Autodesk Inventor part; units mm, degrees
ref_plane "YZ Plane" through (0, 0, 0) normal (1, 0, 0) x (0, 1, 0)
ref_plane "XZ Plane" through (0, 0, 0) normal (0, 1, 0) x (-1, 0, 0)
ref_plane "XY Plane" through (0, 0, 0) normal (0, 0, 1) x (1, 0, 0)
sketch "Boceto1" plane through (0, 0, 0) normal (0, 0, 1) x (1, 0, 0)
  line L0 (-49.9, -20) -> (-45, -20)
  line L1 (-47.8393, -13.9) -> (-45, -13.9)
  line L2 (-50.5, -16.5607) -> (-47.8393, -13.9)
  line L3 (-50.5, -18.2) -> (-50.5, -16.5607)
  line L4 (-48.1, -18.2) -> (-50.5, -18.2)
  line L5 (-49.9, -20) -> (-48.1, -18.2)
  line L6 (-55, -20) -> (-45, -20)
  line L7 (-55, -5.1) -> (-55, -20)
  line L8 (-53.2, -13.1) -> (-55, -14.9)
  line L9 (-53.2, -15.5) -> (-53.2, -13.1)
  line L10 (-51.5606, -15.5) -> (-48.9, -12.8393)
  line L11 (-48.9, -7.1607) -> (-48.9, -12.8393)
  circle A0 centre (-45, -10) radius 2.1
  line L12 (-47.8393, -6.1) -> (-51.2393, -2.7)
  line L13 (-51.5607, -4.5) -> (-48.9, -7.1607)
  line L14 (-53.2, -4.5) -> (-51.5607, -4.5)
  line L15 (-51.2393, -2.7) -> (-53.2, -2.7)
  line L16 (-53.2, -6.9) -> (-53.2, -4.5)
  line L17 (-55, -5.1) -> (-53.2, -6.9)
  line L18 (-51.5606, -15.5) -> (-53.2, -15.5)
  line L19 (-35, 0) -> (-55, 0) construction
  line L20 (-53.2, 0) -> (-53.2, -4.5)
  line L21 (-55, 0) -> (-55, -5.1)
  line L22 (-45, 0) -> (-45, -20) construction
  line L23 (-45, -6.1) -> (-47.8393, -6.1)
  line L24 (-40.1, -20) -> (-45, -20)
  line L25 (-42.1606, -13.9) -> (-45, -13.9)
  line L26 (-39.5, -16.5607) -> (-42.1606, -13.9)
  line L27 (-39.5, -18.2) -> (-39.5, -16.5607)
  line L28 (-41.9, -18.2) -> (-39.5, -18.2)
  line L29 (-40.1, -20) -> (-41.9, -18.2)
  line L30 (-35, -20) -> (-45, -20)
  line L31 (-35, -5.1) -> (-35, -20)
  line L32 (-36.8, -13.1) -> (-35, -14.9)
  line L33 (-36.8, -15.5) -> (-36.8, -13.1)
  line L34 (-38.4393, -15.5) -> (-41.1, -12.8393)
  line L35 (-41.1, -7.1607) -> (-41.1, -12.8393)
  line L36 (-42.1606, -6.1) -> (-38.7607, -2.7)
  line L37 (-38.4393, -4.5) -> (-41.1, -7.1607)
  line L38 (-36.8, -4.5) -> (-38.4393, -4.5)
  line L39 (-38.7607, -2.7) -> (-36.8, -2.7)
  line L40 (-36.8, -6.9) -> (-36.8, -4.5)
  line L41 (-35, -5.1) -> (-36.8, -6.9)
  line L42 (-38.4393, -15.5) -> (-36.8, -15.5)
  line L43 (-36.8, 0) -> (-36.8, -4.5)
  line L44 (-35, 0) -> (-35, -5.1)
  line L45 (-45, -6.1) -> (-42.1606, -6.1)
  line L46 (-49.9, 20) -> (-45, 20)
  line L47 (-47.8393, 13.9) -> (-45, 13.9)
  line L48 (-50.5, 16.5607) -> (-47.8393, 13.9)
  line L49 (-50.5, 18.2) -> (-50.5, 16.5607)
  line L50 (-48.1, 18.2) -> (-50.5, 18.2)
  line L51 (-49.9, 20) -> (-48.1, 18.2)
  line L52 (-55, 20) -> (-45, 20)
  line L53 (-55, 5.1) -> (-55, 20)
  line L54 (-53.2, 13.1) -> (-55, 14.9)
  line L55 (-53.2, 15.5) -> (-53.2, 13.1)
  line L56 (-51.5606, 15.5) -> (-48.9, 12.8393)
  line L57 (-48.9, 7.1607) -> (-48.9, 12.8393)
  circle A1 centre (-45, 10) radius 2.1
  line L58 (-47.8393, 6.1) -> (-51.2393, 2.7)
  line L59 (-51.5607, 4.5) -> (-48.9, 7.1607)
  line L60 (-53.2, 4.5) -> (-51.5607, 4.5)
  line L61 (-51.2393, 2.7) -> (-53.2, 2.7)
  line L62 (-53.2, 6.9) -> (-53.2, 4.5)
  line L63 (-55, 5.1) -> (-53.2, 6.9)
  line L64 (-51.5606, 15.5) -> (-53.2, 15.5)
  line L65 (-53.2, 0) -> (-53.2, 4.5)
  line L66 (-55, 0) -> (-55, 5.1)
  line L67 (-45, 0) -> (-45, 20) construction
  line L68 (-45, 6.1) -> (-47.8393, 6.1)
  line L69 (-40.1, 20) -> (-45, 20)
  line L70 (-42.1606, 13.9) -> (-45, 13.9)
  line L71 (-39.5, 16.5607) -> (-42.1606, 13.9)
  line L72 (-39.5, 18.2) -> (-39.5, 16.5607)
  line L73 (-41.9, 18.2) -> (-39.5, 18.2)
  line L74 (-40.1, 20) -> (-41.9, 18.2)
  line L75 (-36.8, 13.1) -> (-35, 14.9)
  line L76 (-36.8, 15.5) -> (-36.8, 13.1)
  line L77 (-38.4393, 15.5) -> (-36.8, 15.5)
  line L78 (-35, 20) -> (-45, 20)
  line L79 (-35, 5.1) -> (-35, 20)
  line L80 (-38.4393, 15.5) -> (-41.1, 12.8393)
  line L81 (-41.1, 7.1607) -> (-41.1, 12.8393)
  line L82 (-45, 6.1) -> (-42.1606, 6.1)
  line L83 (-38.4393, 4.5) -> (-41.1, 7.1607)
  line L84 (-36.8, 4.5) -> (-38.4393, 4.5)
  line L85 (-42.1606, 6.1) -> (-38.7607, 2.7)
  line L86 (-38.7607, 2.7) -> (-36.8, 2.7)
  line L87 (-36.8, 0) -> (-36.8, 4.5)
  line L88 (-35, 0) -> (-35, 5.1)
  line L89 (-35, 5.1) -> (-36.8, 6.9)
  line L90 (-36.8, 6.9) -> (-36.8, 4.5)
  point P0 (0, 0)
  point P1 (-45, -10)
  point P2 (-45, -10)
  point P3 (-45, 10)
  point P4 (-45, 10)
extrude "Extrusión1" add sketch "Boceto1" along normal blind 400 contours L6 L7 L8 L9 L18 L10 L11 L13 L14 L20 L15 L12 L23 L45 L36 L39 L43 L38 L37 L35 L34 L42 L33 L32 L31 L30 L29 L28 L27 L26 L25 L1 L2 L3 L4 L5 | L21 L66 L63 L62 L65 L20 L16 L17 | L41 L40 L43 L87 L90 L89 L88 L44 | L53 L52 L51 L50 L49 L48 L47 L70 L71 L72 L73 L74 L78 L79 L75 L76 L77 L80 L81 L83 L84 L87 L86 L85 L82 L68 L58 L61 L65 L60 L59 L57 L56 L64 L55 L54
ref_plane "Plano de trabajo1" through (-45, 5.1, 400) normal (1, 0, 0) x (0, 0, -1)
properties part number "Barra"
CAD build for the part. Positions are in the model's coordinates, mm. Give positions to 0.01 mm unless a question says otherwise; leave off trailing zeros.
(1) Drill centre lines: L1, parallel to Y at x = -45, z = 234.5; L2, parallel to Y at x = -36, z = 243; L3, parallel to X at y = -1, z = 345. Where is each one in solid material? Low to high.
(2) Saw through at A-A, the plane z = 157.5. State how many separate pieces and enclosed holes the cut face has, then the cut area to 3 significant figures.
(3) Flat gauge pins, fed straight in: pin 1 (3 mm diameter, centred on x = -44, z = 112, fed in from -Y); pin 2 (0.7 mm diameter, centred on y = -14.5, z = 160.5, fed in from -X); pin 3 (4.5 mm diameter, centred on y = -9, z = 251.5, fed in from +X). Where does each tip first touch, or does it go through?
Results found:
1. L1: y = -13.9 to -12.1, -7.9 to -6.1, 6.1 to 7.9, 12.1 to 13.9
1. L2: y = -20 to -13.9, -6.1 to 6.1, 13.9 to 20
1. L3: x = -55 to -53.2, -36.8 to -35
2. separate pieces: 1
2. enclosed holes: 3
2. area: 294 mm2
3. pin 1: stops at y = -13.9
3. pin 2: stops at x = -54.95
3. pin 3: stops at x = -36.65
